Source: three-view drawing plus pictorial views. Frame: mm from the lowest corner of the part. A direction names the side the tool comes from. Give positions to 0.01 mm unless a question says otherwise; leave off trailing zeros. Loops run counter-clockwise (first coordinate to the right, second up) from the corner with the lowest first, then second, coordinate; pieces in that order, holes last. Notation, with made-up numbers: (61, 31.25) - (120, 31.25) arc R16 cw to (120, 45.25) - close; hole circle Ø7 at (25, 57.5). An arc over 180 degrees is marked (long way). Answer as a JSON object with one key per item and string values. Group by question number.
(1) Access query for the marked faces 1 and 2. Directions: +Z, -Z, +X, -X, +Y, -Y. A direction counts if a zero-diameter tool reaches every point of the face in a straight line with its end or side. Return the directions, or none.
(2) Section query A-A (y = 29). Return loops of the section in (x, z), plus the area to 3 significant figures.
(3) Pin query (flat end, axial travel): P1, Ø4, axis at x = 34.5, y = 7, coming from the +Z side; P2, Ø8, axis at y = 38.5, z = 19.5, coming from the -X side; P3, Ø5, axis at x = 25.5, z = 19.5, coming from the -Y side; P4, Ø9, axis at x = 28, y = 29, coming from the -Z side. Return the tip coordinate at first contact, or that it passes through.
(4) Section query D-D (z = 22.5). Return loops of the section in (x, y).
(5) Material intervals for L1, parallel to Y at x = 29, z = 1; L2, parallel to Z at x = 19, y = 15.5; L3, parallel to X at y = 14, z = 17.5, sorted ascending.
(6) Section query C-C (z = 57.5). Return loops of the section in (x, y).
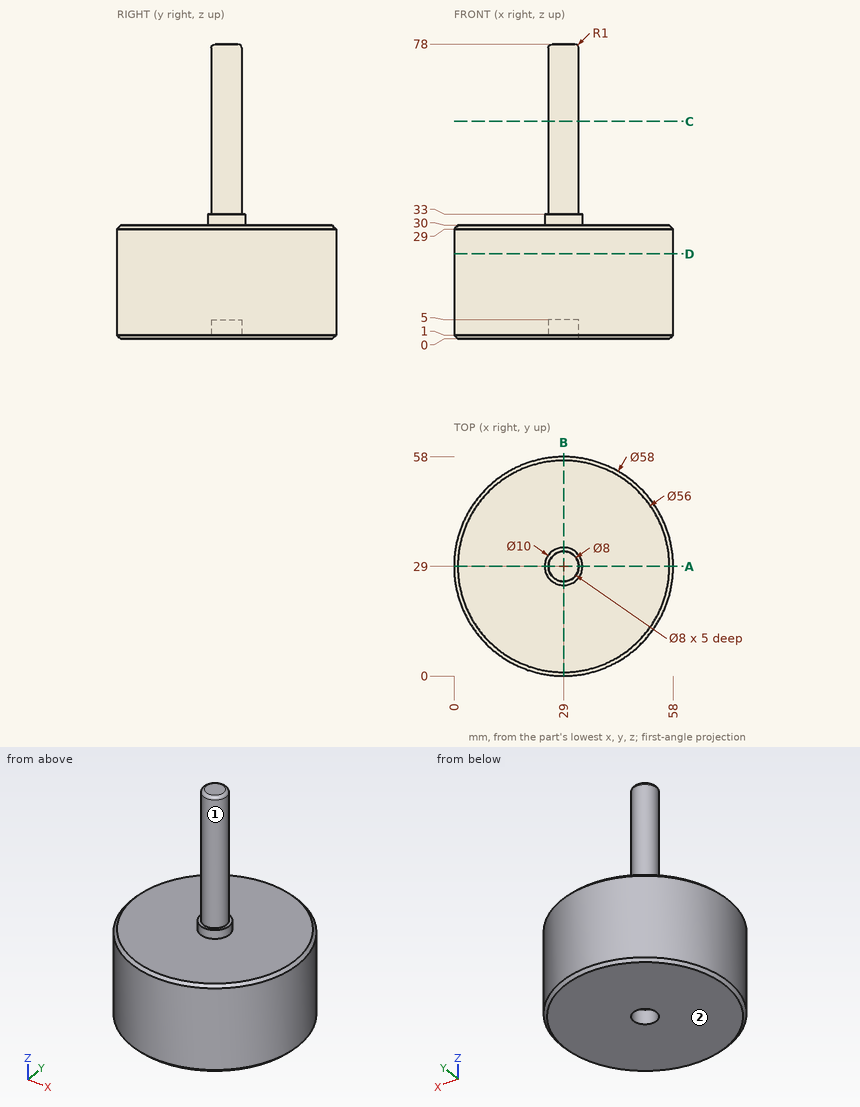
Recorded:
{
 "1": {"face 1": "+Z", "face 2": "-Z, +X, -X, +Y, -Y"},
 "2": {"outline": "(0, 1) - (1, 0) - (25, 0) - (25, 5) - (33, 5) - (33, 0) - (57, 0) - (58, 1) - (58, 29) - (57, 30) - (34, 30) - (34, 33) - (33, 33) - (33, 77) arc R1 ccw to (32, 78) - (26, 78) arc R1 ccw to (25, 77) - (25, 33) - (24, 33) - (24, 30) - (1, 30) - (0, 29) - close", "area": "2,090 mm^2"},
 "3": {"P1": "stops at z = 30", "P2": "stops at x = 0.53", "P3": "stops at y = 0.02", "P4": "stops at z = 0"},
 "4": {"outline": "circle Ø58 at (29, 29)"},
 "5": {"L1": "y = 0 to 25, 33 to 58", "L2": "z = 0 to 30", "L3": "x = 4.18 to 53.82"},
 "6": {"outline": "circle Ø8 at (29, 29)"}
}
